Design review of the part built by this model. Coordinates are the model's own, in mm. Give positions to 0.01 mm unless a question says otherwise; leave off trailing zeros. Loops run counter-clockwise (first coordinate to the right, second up) from the corner with the lowest first, then second, coordinate; pieces in that order, holes last. Notation, with made-up numbers: (-22, -22) - (-8, -22) arc R7 ccw to (-8, -14) - close; hole circle Ø2 at (30.25, -27). An arc over 180 degrees is marked (long way). Write each question's results on one line, items separated by ' | '.
Autodesk Inventor part; units mm, degrees
ref_plane "Work Plane1" through (0, 0, 38.1) normal (0, 0, 1) x (1, 0, 0)
ref_plane "YZ Plane" through (0, 0, 0) normal (1, 0, 0) x (0, 1, 0)
ref_plane "XZ Plane" through (0, 0, 0) normal (0, 1, 0) x (-1, 0, 0)
sketch "Sketch1" plane through (0, 0, 0) normal (0, 0, 1) x (1, 0, 0)
  line L0 (0, 0) -> (-31.75, 0)
  line L1 (-31.75, 0) -> (-31.75, 1.5875)
  line L2 (-31.75, 1.5875) -> (0, 1.5875)
  line L3 (0, 1.5875) -> (0, 0)
  circle A0 centre (0, 4.7625) radius 4.7625
  circle A1 centre (0, 4.7625) radius 3.175
  dimension "d0" = 31.75
  dimension "d1" = 1.5875
  dimension "d2" = 9.525
  dimension "d3" = 6.35
extrude "Extrusion1" add sketch "Sketch1" along normal mid plane 127
ref_plane "Work Plane1" through (0, 0, 38.1) normal (0, 0, 1) x (1, 0, 0)
sketch "Sketch2" plane through (0, 0, 38.1) normal (0, 0, 1) x (1, 0, 0)
  arc A0 (0, 0) -> (-3.5498, 1.5875) centre (0, 4.7625) ccw
  line L0 (-3.5498, 1.5875) -> (-3.5498, 0)
  line L1 (-3.5498, 0) -> (0, 0)
extrude "Extrusion2" cut sketch "Sketch2" against normal blind 25.4
pattern_linear "Rectangular Pattern1" count 2 spacing 50.8 along (0, 0, -1) of "Extrusion2"
sketch "Sketch3" plane through (-31.75, 1.5875, -63.5) normal (0, 1, 0) x (1, 0, 0)
  line L0 (28.2002, 0) -> (0, 0) construction
  line L1 (0, -127) -> (28.2002, -127) construction
  line L2 (0, 0) -> (28.2002, 0) construction
  line L3 (28.2002, 0) -> (28.2002, -127) construction
  line L4 (28.2002, -127) -> (0, -127) construction
  line L5 (0, -127) -> (0, 0) construction
  line L6 (21.8502, -120.65) -> (21.8502, -6.35) construction
  line L7 (21.8502, -6.35) -> (6.35, -6.35) construction
  line L8 (6.35, -6.35) -> (6.35, -120.65) construction
  line L9 (6.35, -120.65) -> (21.8502, -120.65) construction
  line L10 (6.35, -82.55) -> (21.8502, -82.55) construction
  line L11 (6.35, -44.45) -> (21.8502, -44.45) construction
  line L12 (6.35, -6.35) -> (21.8502, -6.35) construction
  point P0 (31.75, -63.5)
  dimension "d12" = 6.35
  dimension "d15" = 114.3
hole "Hole1" at (-9.8998, 1.5875, -57.15) at (-25.4, 1.5875, 57.15) at (-9.8998, 1.5875, 19.05) at (-25.4, 1.5875, -19.05) direction (0, -1, 0) diameter 3.175 end through all
chamfer "Chamfer1" distance 0.7937 angle 45 4 edges at (-25.4, 1.5875, 55.5625) (-9.8998, 1.5875, 17.4625) (-25.4, 1.5875, -20.6375) (-9.8998, 1.5875, -58.7375)
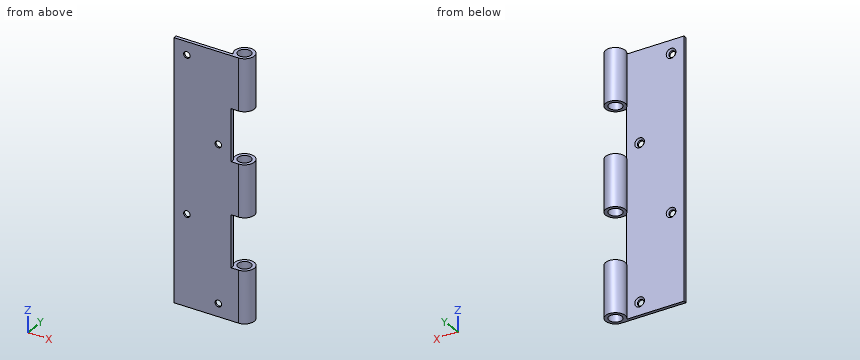
(1) Wall thickness on line 1 along Z through (x, y) = (1, 1); line 2 along Z through (x, y) = (-25.4, 0.6); line 3 along Y through (x, z) = (0, 56.5) (1 decimal): over which ranges is each line inside the solid? List them lowest first. Write a range as from..to.
Answers below:
line 1: -63.5..-38.1, -12.7..12.7, 38.1..63.5 | line 2: -63.5..-20.64, -17.46..55.56, 58.74..63.5 | line 3: 0..1.6, 7.9..9.5
(2) Take a section at C-C on z = -19.05. Give the boundary of the cut face in (x, y).
Answers below:
outline: (-31.75, 0) - (-26.99, 0) - (-26.99, 0.79) - (-27.78, 1.59) - (-31.75, 1.59) - close; (-23.81, 0) - (-3.55, 0) - (-3.55, 1.59) - (-23.02, 1.59) - (-23.81, 0.79) - close
(3) Take a section at A-A on z = -57.15. Count the separate pieces of the cut face and the enclosed holes in it, plus the area to 3 significant figures.
Answers below:
separate pieces: 2 | enclosed holes: 1 | area: 80.4 mm2
(4) Insertion check: P1, Ø1.7, axis at y = 1, z = 20.5, coming from the +X side; P2, Ø1, axis at y = 7, z = -12.5, coming from the +X side; P3, Ø5, axis at x = -11.5, z = 18, coming from the +Y side; P4, Ø10, axis at x = -22.5, z = 21, coming from the -Y side. Each pin has a flat end and moves straight along its axis. Give the tip position at first contact, or say it passes through.
Answers below:
P1: x = -3.55 | P2: x = 4.43 | P3: y = 1.59 | P4: y = 0
(5) Take a section at B-B on x = -25.4. Give the boundary of the cut face in (y, z).
Answers below:
outline: (0, -63.5) - (1.59, -63.5) - (1.59, -21.43) - (0.79, -20.64) - (0, -20.64) - close; (0, -17.46) - (0.79, -17.46) - (1.59, -16.67) - (1.59, 54.77) - (0.79, 55.56) - (0, 55.56) - close; (0, 58.74) - (0.79, 58.74) - (1.59, 59.53) - (1.59, 63.5) - (0, 63.5) - close
